Build history of the part. All positions in model axes, mm. A direction names the side the tool comes from. Round coordinates to 2 decimals unless told otherwise and drop trailing zeros. Write each loop counter-clockwise with the first axis right and the second up, starting at its lowest first coordinate (ties: lowest second). Pieces come first, ordered by that corner, then holes. Notation, with made-up numbers: (80.25, -33.5) - (132.25, -33.5) arc R13 ccw to (132.25, -23.5) - close; hole circle Ø9 at (76, 53). An arc over 180 degrees is marked (long way). Write each question's results on one line, items separated by ' | '.
from build123d import *

# Parameters (mm, degrees)
SKETCH1_W           = 127.25
SKETCH1_H           = 85.15
BOSS_EXTRUDE1_DEPTH = 3.175
SKETCH2_R           = 6.35
CUT_EXTRUDE1_DEPTH  = 4.175
SKETCH3_R           = 7.62
SKETCH3_R_2         = 6.35
CUT_EXTRUDE2_DEPTH  = 4.175
CUT_EXTRUDE3_DEPTH  = 4.175


with BuildPart() as part:
    # Sketch1 → Boss-Extrude1 (new body)
    with BuildSketch(Plane(origin=(0, 0, 0), x_dir=(1, 0, 0), z_dir=(0, 1, 0))):
        with Locations((-63.625, 42.575)):
            Rectangle(SKETCH1_W, SKETCH1_H)
    extrude(amount=BOSS_EXTRUDE1_DEPTH)

    # Sketch2 → Cut-Extrude1 (cut, through all)
    with BuildSketch(Plane(origin=(0, 3.175, 0), x_dir=(1, 0, 0), z_dir=(0, 1, 0))):
        with Locations((-16.925, 71.525)):
            Circle(SKETCH2_R)
    extrude(amount=-CUT_EXTRUDE1_DEPTH, mode=Mode.SUBTRACT)

    # Sketch3 → Cut-Extrude2 (cut, through all)
    with BuildSketch(Plane(origin=(0, 0, 0), x_dir=(-1, 0, 0), z_dir=(0, -1, 0))):
        with Locations((113.425, 71.525)):
            Circle(SKETCH3_R)
        with Locations((113.425, 13.625)):
            Circle(SKETCH3_R)
        with Locations((94.125, 52.225)):
            Circle(SKETCH3_R_2)
        with Locations((55.525, 52.225)):
            Circle(SKETCH3_R)
        with Locations((36.225, 32.925)):
            Circle(SKETCH3_R_2)
    extrude(amount=-CUT_EXTRUDE2_DEPTH, mode=Mode.SUBTRACT)

    # Sketch4 → Cut-Extrude3 (cut, through all)
    with BuildSketch(Plane(origin=(0, 3.175, 0), x_dir=(1, 0, 0), z_dir=(0, 1, 0))):
        with BuildLine():
            Line((-18.195, 13.625), (-18.195, 57.914006297))
            ThreePointArc((-18.195, 57.914006297), (-16.925, 59.184006297), (-15.655, 57.914006297))
            Line((-15.655, 57.914006297), (-15.655, 13.625))
            ThreePointArc((-15.655, 13.625), (-16.925, 12.355), (-18.195, 13.625))
        make_face()
        with BuildLine():
            Line((-36.225, 70.255), (-94.125, 70.255))
            ThreePointArc((-94.125, 70.255), (-95.395, 71.525), (-94.125, 72.795))
            Line((-94.125, 72.795), (-36.225, 72.795))
            ThreePointArc((-36.225, 72.795), (-34.955, 71.525), (-36.225, 70.255))
        make_face()
        with BuildLine():
            Line((-114.695, 25.905281506), (-114.695, 57.683208878))
            ThreePointArc((-114.695, 57.683208878), (-113.425, 58.953208878), (-112.155, 57.683208878))
            Line((-112.155, 57.683208878), (-112.155, 25.905281506))
            ThreePointArc((-112.155, 25.905281506), (-113.425, 24.635281506), (-114.695, 25.905281506))
        make_face()
        with BuildLine():
            Line((-36.225, 14.895), (-94.125, 14.895))
            ThreePointArc((-94.125, 14.895), (-95.395, 13.625), (-94.125, 12.355))
            Line((-94.125, 12.355), (-36.225, 12.355))
            ThreePointArc((-36.225, 12.355), (-34.955, 13.625), (-36.225, 14.895))
        make_face()
    extrude(amount=-CUT_EXTRUDE3_DEPTH, mode=Mode.SUBTRACT)


solid = part.part
(1) Slice it at A-A, the plane x = -69.5. Write the cut outline in (y, z) (3 decimals).
Worked answers:
outline: (0, -85.15) - (3.175, -85.15) - (3.175, -72.795) - (0, -72.795) - close; (0, -70.255) - (3.175, -70.255) - (3.175, -14.895) - (0, -14.895) - close; (0, -12.355) - (3.175, -12.355) - (3.175, 0) - (0, 0) - close
(2) Two-plate mould, pull along Z, no slides. Class faces 3 (the cylindrical face through (-107.809, 1.565, -76.675)), 4 (the cylindrical face through (-113.453, 1.61, -58.953)), 5 (the flat face through (-65, 2, -85.15)), 6 (the flat face through (-127.25, 2, -42)): released by +Z, released by -Z, zero draft, split by the parting line, or undercut.
Worked answers:
face 3: undercut | face 4: undercut | face 5: released by -Z | face 6: zero draft
(3) Flat gauge pins, fed straight in: pin 1 Ø14.5 at (x, z) = (-36.225, -32.925) entering from -Y; pin 2 Ø12 at (x, z) = (-55.525, -52.225) entering from +Y. Where does each tip first touch, or does it go through?
Worked answers:
pin 1: stops at y = 0 | pin 2: passes through
(4) Drill centre lines: probe 1 along Z at (x, y) = (-47, 1.05) (3 decimals); probe 2 along Z at (x, y) = (-61, 2.1) (3 decimals); probe 3 along Z at (x, y) = (-37.5, 1.1) (3 decimals). Where is each one in solid material? Low to high. Write a range as [from, to].
Worked answers:
probe 1: z = [-85.15, -72.795], [-70.255, -14.895], [-12.355, 0] | probe 2: z = [-85.15, -72.795], [-70.255, -57.525], [-46.925, -14.895], [-12.355, 0] | probe 3: z = [-85.15, -72.795], [-70.255, -39.146], [-26.704, -14.895], [-12.355, 0]
(5) Slice it at C-C, the plane z = -55. Write the cut outline in (x, y) (3 decimals).
Worked answers:
outline: (-127.25, 0) - (-114.695, 0) - (-114.695, 3.175) - (-127.25, 3.175) - close; (-112.155, 0) - (-99.837, 0) - (-99.837, 3.175) - (-112.155, 3.175) - close; (-88.413, 0) - (-62.622, 0) - (-62.622, 3.175) - (-88.413, 3.175) - close; (-48.428, 0) - (-18.195, 0) - (-18.195, 3.175) - (-48.428, 3.175) - close; (-15.655, 0) - (0, 0) - (0, 3.175) - (-15.655, 3.175) - close
(6) Slice it at D-D, the plane x = -39. Write the cut outline in (y, z) (3 decimals).
Worked answers:
outline: (0, -85.15) - (3.175, -85.15) - (3.175, -72.795) - (0, -72.795) - close; (0, -70.255) - (3.175, -70.255) - (3.175, -38.637) - (0, -38.637) - close; (0, -27.213) - (3.175, -27.213) - (3.175, -14.895) - (0, -14.895) - close; (0, -12.355) - (3.175, -12.355) - (3.175, 0) - (0, 0) - close
(7) Slice it at B-B, the plane z = -67. Write the cut outline in (x, y) (3 decimals), and give its area (3 significant figures).
Worked answers:
outline: (-127.25, 0) - (-119.556, 0) - (-119.556, 3.175) - (-127.25, 3.175) - close; (-107.294, 0) - (-21.38, 0) - (-21.38, 3.175) - (-107.294, 3.175) - close; (-12.47, 0) - (0, 0) - (0, 3.175) - (-12.47, 3.175) - close | area: 337 mm2
(8) Tool access for faces 1 (the cylindrical face through (-34.955, 1.61, -13.597)), 2 (the flat face through (-65, 3.175, -43)): list every direction of +Z, -Z, +X, -X, +Y, -Y with a clear straight run to the whole face (end or side of a thin tool).
Worked answers:
face 1: +Y, -Y | face 2: +Z, -Z, +X, -X, +Y
